The listing builds one solid part. Answer for the finished solid, in the listing's coordinates (mm). A direction names the side the tool comes from. Coordinates: 2 decimals unless noted, no trailing zeros. Order: outer loops, then holes, each group sorted by start corner. A loop starts at its lowest first (then second) coordinate and runs counter-clockwise, first axis right, second up. Notation, with made-up numbers: (26, -22) - (38, -22) arc R14 ccw to (38, -4) - close; hole circle Ø7 at (40, 74.5). An arc over 180 degrees is marked (long way). Use a Markdown table: item, result. Add a question column.
Item 1: The part is cut by section A-A, the plane y = 8. Give the vertices of the cut face in (x, z), then the cut area to 3 significant figures.
Item 2: The part is cut by section D-D, the plane z = -8. Give the vertices of the cut face in (x, y).
Item 3: Flat-ended cylindrical pins translate along their axes: P1, Ø4, axis at y = 12, z = -0.5, coming from the +X side; P2, Ø4, axis at y = 11, z = -1.5, coming from the -X side; P3, Ø3, axis at x = 1, y = 14, coming from the -Z side. Find the tip coordinate at first contact, or state that the pin passes through.
Item 4: For faces 1 (the cylindrical face through (4.949, 10.902, -4.965)), 2 (the cylindrical face through (4.214, 0.986, 0.553)), 3 (the cylindrical face through (4.949, 10.902, 4.965)), determine the directions among +Z, -Z, +X, -X, +Y, -Y from which every point of the face is accessible in a straight line to the end or side of a thin tool.
Item 5: The part is cut by section B-B, the plane z = 0. Give the vertices of the cut face in (x, y).
Item 6: The mould has two halves that part along Z. Classify faces 4 (the cylindrical face through (-6.81, 1.52, -0.16)), 5 (the cylindrical face through (-4.965, 10.902, 4.949)), 6 (the cylindrical face through (-4.965, 10.902, -4.949)): released by +Z, released by -Z, zero draft, split by the parting line, or undercut.
Item 7: Find the intervals of material crossed by line 1 along X through (y, z) = (1.4, 0); line 2 along X through (y, z) = (10.75, 0); line 3 along X through (y, z) = (1.15, 8), in increasing order.
Item 8: The part is cut by section C-C, the plane x = 0. State how many separate pieces and enclosed holes the cut face has, then the cut area to 3 significant figures.
from build123d import *

# Parameters (mm, degrees)
SKETCH1_W           = 7.2361
SKETCH1_H           = 3
BOSS_EXTRUDE1_START = 15
SKETCH7_W           = 10.5
SKETCH7_H           = 10.5
SKETCH7_R           = 3.2639
BOSS_EXTRUDE1_DEPTH = 15
SKETCH3_R           = 1.7
CUT_EXTRUDE1_DEPTH  = 33.886404519
SKETCH4_R           = 1.2
CUT_EXTRUDE2_DEPTH  = 22.10687099
FILLET1_R           = 1
FILLET2_R           = 1
SKETCH8_R           = 4.25
CUT_EXTRUDE3_DEPTH  = 3
FILLET3_R           = 1


with BuildPart() as part:
    # Sketch1 → Revolve1 (revolve)
    with BuildSketch(Plane.XY, mode=Mode.PRIVATE) as revolve1_sk:
        with Locations((6.88195, 1.5)):
            Rectangle(SKETCH1_W, SKETCH1_H)
    revolve(revolve1_sk.sketch.rotate(Axis((0, 0, 0), (0, 1, 0)), 90), axis=Axis((0, 0, 0), (0, 1, 0)))

    # Sketch7 → Boss-Extrude1 (add)
    with BuildSketch(Plane(origin=(0, 3, 0), x_dir=(1, 0, 0), z_dir=(0, 1, 0)).offset(BOSS_EXTRUDE1_START)):
        Rectangle(SKETCH7_W, SKETCH7_H)
        with Locations(Location((0, 0, 0), (0, 0, 90))):
            Circle(SKETCH7_R, mode=Mode.SUBTRACT)
    extrude(amount=-BOSS_EXTRUDE1_DEPTH)

    # Sketch3 → Cut-Extrude1 (cut, through all)
    with BuildSketch(Plane(origin=(12.071067812, 0, 5.25), x_dir=(-1, 0, 0), z_dir=(0, 0, -1))):
        with Locations(Location((12.071067812, 8, 0), (0, 0, 180))):
            Circle(SKETCH3_R)
    extrude(amount=CUT_EXTRUDE1_DEPTH, mode=Mode.SUBTRACT)

    # Sketch4 → Cut-Extrude2 (cut, through all)
    with BuildSketch(Plane(origin=(0, 3, 0), x_dir=(1, 0, 0), z_dir=(0, 1, 0))):
        with Locations(Location((0, 8, 0), (0, 0, 270))):
            Circle(SKETCH4_R)
        with Locations(Location((8, 0, 0), (0, 0, 270))):
            Circle(SKETCH4_R)
        with Locations(Location((0, -8, 0), (0, 0, 270))):
            Circle(SKETCH4_R)
        with Locations(Location((-8, 0, 0), (0, 0, 270))):
            Circle(SKETCH4_R)
    extrude(amount=-CUT_EXTRUDE2_DEPTH, mode=Mode.SUBTRACT)

    # Fillet1
    fillet1_edges = [part.edges().sort_by_distance(p)[0] for p in [
        (5.25, 10.5, 5.25),
        (5.25, 10.5, -5.25),
        (-5.25, 10.5, -5.25),
        (-5.25, 10.5, 5.25),
    ]]
    fillet(fillet1_edges, radius=FILLET1_R)

    # Fillet2
    fillet2_edges = [part.edges().sort_by_distance(p)[0] for p in [
        (0, 3, -5.25),
        (5.25, 3, 0),
        (-5.25, 3, 0),
        (0, 3, 5.25),
        (4.957106781, 3, -4.957106781),
        (-4.957106781, 3, -4.957106781),
        (4.957106781, 3, 4.957106781),
        (-4.957106781, 3, 4.957106781),
    ]]
    fillet(fillet2_edges, radius=FILLET2_R)

    # Sketch8 → Cut-Extrude3 (cut)
    with BuildSketch(Plane.XZ):
        with Locations(Location((0, 0, 0), (0, 0, 270))):
            Circle(SKETCH8_R)
    extrude(amount=-CUT_EXTRUDE3_DEPTH, mode=Mode.SUBTRACT)

    # Fillet3
    # the kernel refuses this fillet: 1 mm, written as the material it adds along each edge
    with BuildSketch(Plane(origin=(0, 3, 0), x_dir=(0, 0, -1), z_dir=(-1, 0, 0))) as fillet3_piece_1_section:
        with BuildLine():
            CenterArc((4.25 - FILLET3_R, FILLET3_R), FILLET3_R, 270, 90)
            Line((4.25 - FILLET3_R, 0), (4.25, 0))
            Line((4.25, 0), (4.25, FILLET3_R))
        make_face()
    fillet3_piece_1 = revolve(axis=Axis((0, 3, 0), (0, -1, 0)), mode=Mode.PRIVATE)
    fillet3_piece_1 = fillet3_piece_1 - Plane(origin=(0, 2.715239817, 0), x_dir=(0, 0, -1), z_dir=(0, 1, 0)) * Cylinder(3.2639, 17, mode=Mode.PRIVATE)
    add(fillet3_piece_1)


solid = part.part
Solution:
| question | item | result |
|---|---|---|
| 1 | outline | (-5.25, -4.25) arc R1 ccw to (-4.25, -5.25) - (-1.7, -5.25) - (-1.7, -2.79) arc R3.26 cw to (-1.7, 2.79) - (-1.7, 5.25) - (-4.25, 5.25) arc R1 ccw to (-5.25, 4.25) - close; (1.7, -5.25) - (4.25, -5.25) arc R1 ccw to (5.25, -4.25) - (5.25, 4.25) arc R1 ccw to (4.25, 5.25) - (1.7, 5.25) - (1.7, 2.79) arc R3.26 cw to (1.7, -2.79) - close |
| 1 | area | 61.4 mm2 |
| 2 | outline | (-6.8, 0) - (-1.2, 0) - (-1.2, 3) - (-6.8, 3) - close; (1.2, 0) - (6.8, 0) - (6.8, 3) - (1.2, 3) - close |
| 3 | P1 | stops at x = 5.25 |
| 3 | P2 | stops at x = -5.25 |
| 3 | P3 | stops at z = -5.25 |
| 4 | face 1 | -Z, +X, +Y |
| 4 | face 2 | -Y |
| 4 | face 3 | +Z, +X, +Y |
| 5 | outline | (-10.5, 0) - (-9.2, 0) - (-9.2, 3) - (-10.5, 3) - close; (-6.8, 0) - (-4.25, 0) - (-4.25, 2) arc R1 cw to (-3.26, 3) - (-3.26, 18) - (-5.25, 18) - (-5.25, 4) arc R1 cw to (-6.25, 3) - (-6.8, 3) - close; (3.26, 3) arc R1 cw to (4.25, 2) - (4.25, 0) - (6.8, 0) - (6.8, 3) - (6.25, 3) arc R1 cw to (5.25, 4) - (5.25, 18) - (3.26, 18) - close; (9.2, 0) - (10.5, 0) - (10.5, 3) - (9.2, 3) - close |
| 6 | face 4 | undercut |
| 6 | face 5 | released by +Z |
| 6 | face 6 | released by -Z |
| 7 | line 1 | x = -10.5 to -9.2, -6.8 to -4.25, 4.25 to 6.8, 9.2 to 10.5 |
| 7 | line 2 | x = -5.25 to -3.26, 3.26 to 5.25 |
| 7 | line 3 | x = -6.8 to -1.2, 1.2 to 6.8 |
| 8 | separate pieces | 6 |
| 8 | enclosed holes | 0 |
| 8 | area | 70.0 mm2 |
